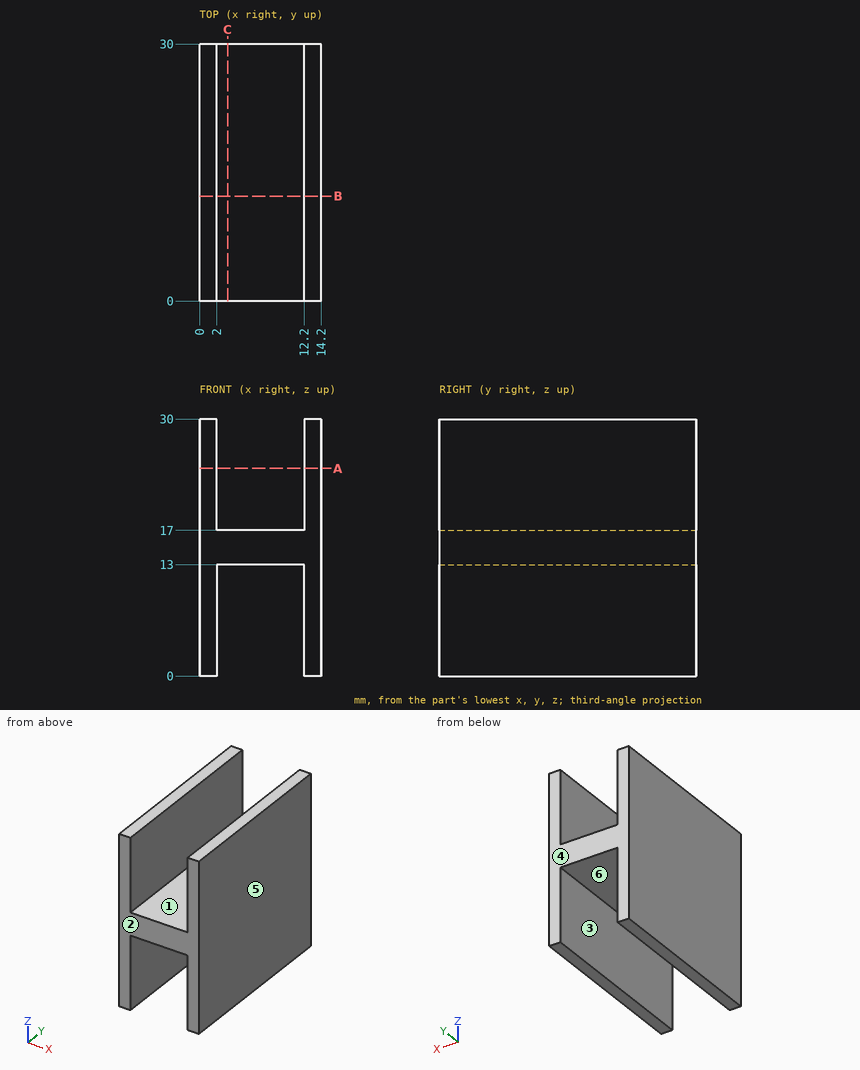
For this review, use the dimensioned drawing (mm, ordinates from the lowest corner) and the shaded views. A direction names the side the tool comes from. Round coordinates to 2 decimals unless told otherwise and drop trailing zeros. Order: outer loops, then holes, each group sorted by start corner. A loop starts at its lowest first (then second) coordinate and runs counter-clockwise, first axis right, second up. Notation, with made-up numbers: (42, 80.25) -> (96, 80.25) arc R25 cw to (96, 117.25) -> close; hole circle Ø2 at (31, 71). An arc over 180 degrees is marked (long way). Use CSV: the item, a comma, the result in double quotes. Start each with the question number.
(1) Mouldability with a two-part tool opening along X and no side actions: class the marked faces 4, 5 and 6 as pulls with the +X half, pulls with the -X half, needs draft (parallel to the pull), parting line crosses it, or undercut.
(2) Wall thickness on probe 1 along X at (y, z) = (22, 26.25); probe 2 along Z at (x, y) = (11.5, 13): over which ranges is each line inside the solid? List them lowest first. Write a range as from..to.
(3) Insertion check: pin 1 (10 mm diameter, centred on y = 21, z = 17, fed in from -X); pin 2 (4 mm diameter, centred on x = 9, y = 17.5, fed in from +Z); pin 3 (2 mm diameter, centred on x = 3.5, z = 22, fed in from -Y). Each pin has a flat end and moves straight along its axis. Give the tip position at first contact, or say it passes through.
(4) Consider section A-A on z = 24.25. Write out the cut boundary in (x, y).
(5) Tool access review of the marked faces 1, 2 and 3: name each direction out of +Z, -Z, +X, -X, +Y, -Y from which nothing blocks a thin tool from reaching the whole face with its end or side.
(6) Consider section B-B on y = 12.25. Write out the cut boundary in (x, z).
(7) Consider section C-C on x = 3.25. Write out the cut boundary in (y, z), and give its area (3 significant figures).
Responses:
1,face 4,"needs draft"
1,face 5,"pulls with the +X half"
1,face 6,"undercut"
2,probe 1,"0..2, 12.2..14.2"
2,probe 2,"13..17"
3,pin 1,"x = 0"
3,pin 2,"z = 17"
3,pin 3,"through"
4,outline,"(0, 0) -> (2, 0) -> (2, 30) -> (0, 30) -> close; (12.2, 0) -> (14.2, 0) -> (14.2, 30) -> (12.2, 30) -> close"
5,face 1,"+Z, +Y, -Y"
5,face 2,"+Z, -Z, +X, -X, -Y"
5,face 3,"-Z, +Y, -Y"
6,outline,"(0, 0) -> (2, 0) -> (2, 13) -> (12.2, 13) -> (12.2, 0) -> (14.2, 0) -> (14.2, 30) -> (12.2, 30) -> (12.2, 17) -> (2, 17) -> (2, 30) -> (0, 30) -> close"
7,outline,"(0, 13) -> (30, 13) -> (30, 17) -> (0, 17) -> close"
7,area,"120 mm²"
